CAD build for the part. Positions are in the model's coordinates, mm. A direction names the side the tool comes from. Give positions to 0.01 mm unless a question says otherwise; leave off trailing zeros. Order: outer loops, then holes, each group sorted by start corner. A loop starts at its lowest first (then second) coordinate and runs counter-clockwise, first axis right, second up.
Item 1: Flat gauge pins, fed straight in: P1, Ø2, axis at y = -9, z = -16, coming from the +X side; P2, Ø12, axis at y = -16, z = -11, coming from the -X side; P3, Ø1.4, axis at x = 6.5, z = -27.5, coming from the +Y side. Where does each tip first touch, or does it go through?
Item 2: Wall check: L1, parallel to Z at x = 5.75, y = -7.5; L2, parallel to Z at x = 5, y = -16; L3, parallel to X at y = -9, z = -11. Give the ranges that are in metal, low to high.
Item 3: Two-plate mould, pull along X, no slides. Class faces 1 (the flat face through (-14.5, -12.54, -27.48)), 2 (the flat face through (-11.454, -12.535, -27.464)), 3 (the flat face through (12, -15.2, -14.9)): released by +X, released by -X, zero draft, split by the parting line, or undercut.
Item 4: Which spindle directions (+Z, -Z, +X, -X, +Y, -Y) get a long thin tool onto all of the face, cutting with end or side? Do faces 4 (the flat face through (6, -23.6, -28)), 5 (the flat face through (-8, -10, -28)), 6 (the flat face through (-8, -13, -28.5)), 7 (the flat face through (6, -15.639, -15)), 8 (the flat face through (-12.654, -12.535, -27.464)). Say none if no direction does.
Item 5: Band-saw the part on B-B on y = -9. Give the cut face in (x, z), plus the area to 3 significant figures.
Item 6: Band-saw the part on C-C on z = -14.5. Give the cut face in (x, y), plus the area to 3 significant figures.
Item 7: Band-saw the part on D-D on x = 6.75. Give the cut face in (y, z), plus the area to 3 significant figures.
Item 8: Band-saw the part on A-A on y = -17. Give the cut face in (x, z), plus the area to 3 significant figures.
```python
from build123d import *

# Parameters (mm, degrees)
BOSS_EXTRUDE1_DEPTH = 30
SKETCH4_W           = 24
SKETCH4_H           = 14
CUT_EXTRUDE2_DEPTH  = 25
SKETCH5_W           = 1.7
SKETCH5_H           = 1.8
CUT_EXTRUDE3_DEPTH  = 15
CUT_EXTRUDE4_DEPTH  = 11
BOSS_EXTRUDE2_DEPTH = 5


with BuildPart() as part:
    # Sketch1 → Boss-Extrude1 (new body)
    with BuildSketch(Plane.XY):
        Polygon((0, 0), (0, -25), (12, -25), (12, -15), (5, 0), align=None)
    extrude(amount=-BOSS_EXTRUDE1_DEPTH)

    # Sketch4 → Cut-Extrude2 (cut)
    with BuildSketch(Plane.ZY):
        with Locations((-15, -22.638599401)):
            Rectangle(SKETCH4_W, SKETCH4_H)
    extrude(amount=-CUT_EXTRUDE2_DEPTH, mode=Mode.SUBTRACT)

    # Sketch5 → Cut-Extrude3 (cut)
    with BuildSketch(Plane.ZY):
        with Locations((-2.15, -22.7)):
            Rectangle(SKETCH5_W, SKETCH5_H)
    cut_extrude3 = extrude(amount=-CUT_EXTRUDE3_DEPTH, mode=Mode.SUBTRACT)

    # Mirror1: Cut-Extrude3 across plane
    add(cut_extrude3.mirror(Plane.XY.offset(-15)), mode=Mode.SUBTRACT)

    # Sketch6 → Cut-Extrude4 (cut, symmetric)
    with BuildSketch(Plane.XY.offset(-15)):
        Polygon((5, 0), (5, -13), (11.066666667, -13), align=None)
    extrude(amount=CUT_EXTRUDE4_DEPTH, both=True, mode=Mode.SUBTRACT)

    # Sketch7 → Boss-Extrude2 (add)
    with BuildSketch(Plane(origin=(0, -15, 0), x_dir=(1, 0, 0), z_dir=(0, 1, 0))):
        Polygon((0, 28.5), (-16, 28.5), (-16, 28), (-14.9, 28), (-14.665549599, 28), (-14.327251213, 26.943471152), (-14.004330027, 26.943471152), (-13.7, 28), (-13.465549599, 28), (-13.127251213, 26.943471152), (-12.804330027, 26.943471152), (-12.5, 28), (-12.265549599, 28), (-11.927251213, 26.943471152), (-11.604330027, 26.943471152), (-11.3, 28), (-11.065549599, 28), (-10.727251213, 26.943471152), (-10.404330027, 26.943471152), (-10.1, 28), (-9.865549599, 28), (-9.527251213, 26.943471152), (-9.204330027, 26.943471152), (-8.9, 28), (-8.665549599, 28), (-8.327251213, 26.943471152), (-8.004330027, 26.943471152), (-7.7, 28), (-7.465549599, 28), (-7.127251213, 26.943471152), (-6.804330027, 26.943471152), (-6.5, 28), (-6.265549599, 28), (-5.927251213, 26.943471152), (-5.604330027, 26.943471152), (-5.3, 28), (-5.065549599, 28), (-4.727251213, 26.943471152), (-4.404330027, 26.943471152), (-4.1, 28), (-3.865549599, 28), (-3.527251213, 26.943471152), (-3.204330027, 26.943471152), (-2.9, 28), (-2.665549599, 28), (-2.327251213, 26.943471152), (-2.004330027, 26.943471152), (-1.7, 28), (-1.465549599, 28), (-1.127251213, 26.943471152), (-0.804330027, 26.943471152), (-0.5, 28), (0, 28), align=None)
    extrude(amount=BOSS_EXTRUDE2_DEPTH)


solid = part.part
```
The answers:
1. P1: stops at x = 5
1. P2: stops at x = 0
1. P3: stops at y = -1.71
2. L1: z = -30 to -26, -4 to 0
2. L2: z = -30 to -27, -3 to 0
2. L3: x = 0 to 5
3. face 1: released by -X
3. face 2: undercut
3. face 3: released by +X
4. face 4: +X, -X
4. face 5: +Z, -Z, -X, +Y
4. face 6: -Z, -X, +Y, -Y
4. face 7: +X, -X, -Y
4. face 8: +Z, +Y, -Y
5. outline: (0, -30) - (9.2, -30) - (9.2, -26) - (5, -26) - (5, -4) - (9.2, -4) - (9.2, 0) - (0, 0) - close
5. area: 184 mm2
6. outline: (0, -15.64) - (12, -15.64) - (12, -15) - (11.07, -13) - (5, -13) - (5, 0) - (0, 0) - close
6. area: 95.7 mm2
7. outline: (-25, -30) - (-3.75, -30) - (-3.75, -26) - (-13, -26) - (-13, -4) - (-3.75, -4) - (-3.75, 0) - (-25, 0) - (-25, -3) - (-23.6, -3) - (-23.6, -1.3) - (-21.8, -1.3) - (-21.8, -3) - (-15.64, -3) - (-15.64, -27) - (-21.8, -27) - (-21.8, -28.7) - (-23.6, -28.7) - (-23.6, -27) - (-25, -27) - close
7. area: 203 mm2
8. outline: (0, -30) - (12, -30) - (12, -27) - (0, -27) - close; (0, -3) - (12, -3) - (12, 0) - (0, 0) - close
8. area: 72.0 mm2
